Drawing for the job (mm, zero at the part's lowest x, y, z). A direction names the side the tool comes from. Round coordinates to 2 decimals unless told otherwise and drop trailing zeros. Loops run counter-clockwise (first coordinate to the right, second up) from the corner with the lowest first, then second, coordinate; pieces in that order, holes last. Notation, with made-up numbers: M -38.5,74.5 L -26.5,74.5 A29 cw -26.5,98.5 Z; hole C 21,35 d1. An arc over 180 degrees is marked long. Write each question's results on one line, items separated by ' | '.
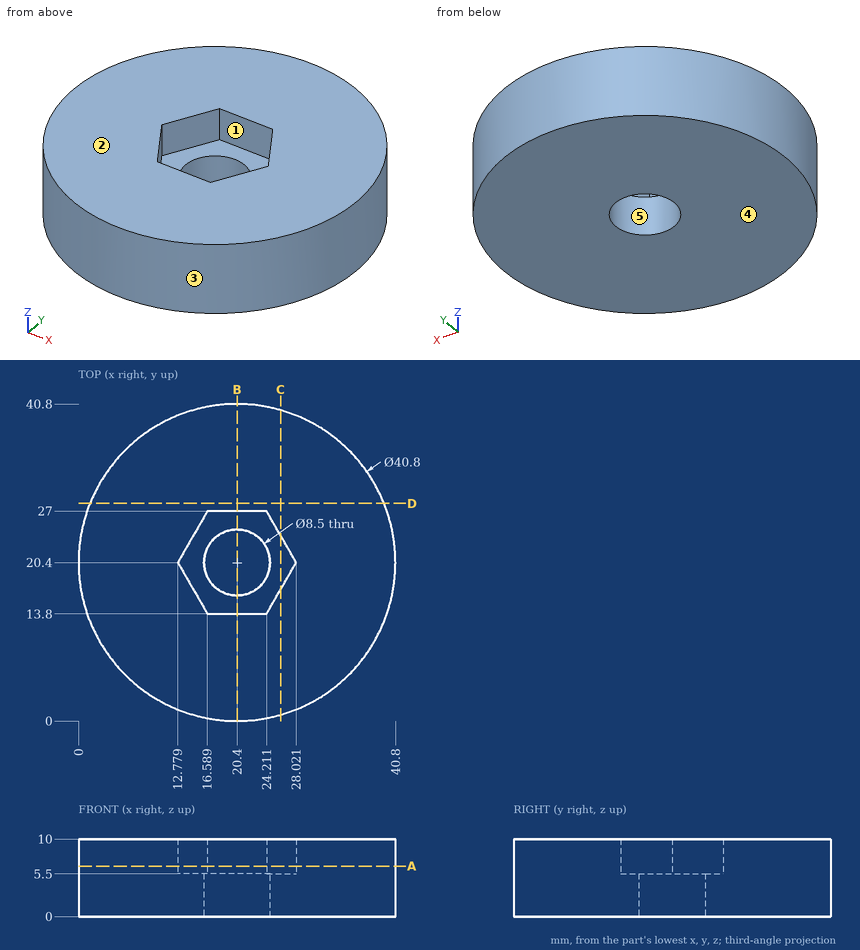
Item 1: Band-saw the part on A-A on z = 6.5. Give the cut face in (x, y), and give its area (3 significant figures).
Filled sheet:
outline: C 20.4,20.4 d40.8; hole M 12.78,20.4 L 16.59,13.8 L 24.21,13.8 L 28.02,20.4 L 24.21,27 L 16.59,27 Z | area: 1,160 mm^2
Item 2: Band-saw the part on B-B on x = 20.4. Give the cut face in (y, z).
Filled sheet:
outline: M 0,0 L 16.15,0 L 16.15,5.5 L 13.8,5.5 L 13.8,10 L 0,10 Z; M 24.65,0 L 40.8,0 L 40.8,10 L 27,10 L 27,5.5 L 24.65,5.5 Z
Item 3: Two-plate mould, pull along Y, no slides. Class the marked faces 3, 4 and 5: +Y half, -Y half, draft (parallel to the pull), parting line (faces both ways), or undercut.
Filled sheet:
face 3: parting line | face 4: draft | face 5: undercut
Item 4: Drop flat-ended pins along their axis: P1, Ø8, axis at x = 23, y = 23.5, coming from the -Z side; P2, Ø1, axis at x = 11.5, z = 7.5, coming from the +Y side; P3, Ø4, axis at y = 14, z = 8, coming from the +X side; P4, Ø6, axis at x = 8.5, z = 4.5, coming from the +Y side (1 decimal). Give the stop position or say it passes through.
Filled sheet:
P1: z = 0 | P2: y = 38.99 | P3: x = 40.32 | P4: y = 38.8
Item 5: Wall check: L1, parallel to Y at x = 20.4, z = 3.8; L2, parallel to Y at x = 25, z = 7 (1 decimal); L3, parallel to Z at x = 18.5, y = 14.5. Give the ranges that are in metal, low to high.
Filled sheet:
L1: 0 to 16.15, 24.65 to 40.8 | L2: 0.5 to 15.2, 25.6 to 40.3 | L3: 0 to 5.5
Item 6: Band-saw the part on C-C on x = 26. Give the cut face in (y, z).
Filled sheet:
outline: M 0.78,0 L 40.02,0 L 40.02,10 L 23.9,10 L 23.9,5.5 L 16.9,5.5 L 16.9,10 L 0.78,10 Z
Item 7: Band-saw the part on D-D on y = 28. Give the cut face in (x, z), and give its area (3 significant figures).
Filled sheet:
outline: M 1.47,0 L 39.33,0 L 39.33,10 L 1.47,10 Z | area: 379 mm^2
Item 8: Which spindle directions (+Z, -Z, +X, -X, +Y, -Y) get a long thin tool onto all of the face, cutting with end or side? Do the marked faces 1 and 2. Say none if no direction does.
Filled sheet:
face 1: +Z | face 2: +Z, +X, -X, +Y, -Y
